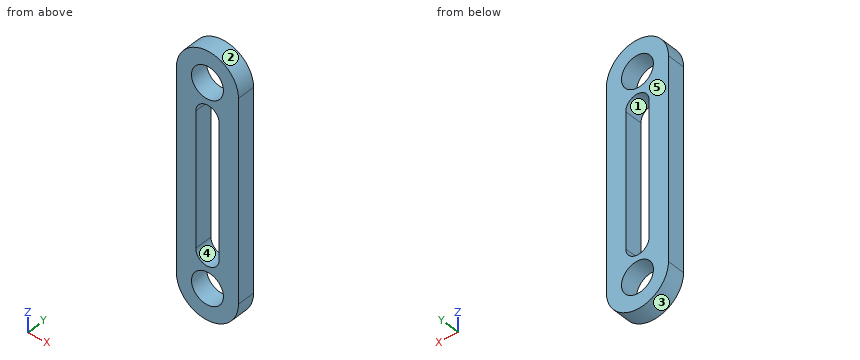
```python
from build123d import *

# Parameters (mm, degrees)
BOSS_EXTRUDE1_DEPTH             = 10
M16_CLEARANCE_HOLE1_D           = 17.5
M16_CLEARANCE_HOLE1_ON_FACE_2_D = 17.5


with BuildPart() as part:
    # Sketch1 → Boss-Extrude1 (new body)
    with BuildSketch(Plane(origin=(0, 0, 0), x_dir=(1, 0, 0), z_dir=(0, 1, 0))):
        with BuildLine():
            Line((17, 0), (17, -110))
            ThreePointArc((17, -110), (0, -127), (-17, -110))
            Line((-17, -110), (-17, 0))
            ThreePointArc((-17, 0), (0, 17), (17, 0))
        make_face()
        with BuildLine():
            Line((-6.39610115, -91.666666667), (-6.39610115, -18.333333333))
            ThreePointArc((-6.39610115, -18.333333333), (0, -11.937232183), (6.39610115, -18.333333333))
            Line((6.39610115, -18.333333333), (6.39610115, -91.666666667))
            ThreePointArc((6.39610115, -91.666666667), (0, -98.062767817), (-6.39610115, -91.666666667))
        make_face(mode=Mode.SUBTRACT)
    extrude(amount=BOSS_EXTRUDE1_DEPTH)

    # M16 Clearance Hole1 (through all)
    with Locations(Plane(origin=(0, 10, 110), x_dir=(0, 0, 1), z_dir=(0, 1, 0))):
        with Locations((0, 0), (-110, 0)):
            Hole(M16_CLEARANCE_HOLE1_D / 2)

    # M16 Clearance Hole1 on face 2 (through all)
    with Locations(Plane(origin=(0, 0, 0), x_dir=(0, 0, -1), z_dir=(0, -1, 0))):
        with Locations((0, 0)):
            Hole(M16_CLEARANCE_HOLE1_ON_FACE_2_D / 2)


solid = part.part
```
Can you work these out from the model? Positions are in its coordinate system, mm. Face numbers are marked on the shaded views. A direction names the side the tool comes from. Round coordinates to 2 decimals unless told otherwise and drop trailing zeros. Order: outer loops, then holes, each group sorted by start corner. A loop starts at its lowest first (then second) coordinate and runs counter-clockwise, first axis right, second up. Notation, with made-up numbers: (-7, -16.75) -> (1, -16.75) arc R8 ccw to (1, -5.75) -> close; hole circle Ø9 at (74, 58.25). An arc over 180 degrees is marked (long way). Return JSON: item names as keys, results as strings. Group by question number.
1. I need wall thicknesses on line 1 (X direction, y = 5.75, z = 52); line 2 (X direction, y = 7.75, z = 110); line 3 (Z direction, x = -4.5, y = 6). Which ranges of each line are inside material? Lowest first, please. Write a range as [from, to].
2. If we section it at A-A, the plane x = 0: Write out the boundary of the cut face in (y, z).
3. If we section it at B-B, the plane z = 89: Write out the boundary of the cut face in (x, y), then the cut area to 3 significant figures.
4. Which directions (+Z, -Z, +X, -X, +Y, -Y) give clear straight access to the entire face, cutting with the end or side of a thin tool? Please do the marked faces 1 and 2.
5. We'd pull the mould along Z, two halves only. Please class the marked faces 3, 4 and 5: released by +Z, released by -Z, zero draft, split by the parting line, or undercut.
6. If we section it at D-D, the plane x = 11.5: Write out the boundary of the cut face in (y, z), then the cut area to 3 significant figures.
7. If we section it at C-C, the plane y = 3.25: Write out the boundary of the cut face in (x, z).
Output values:
{
 "1": {"line 1": "[-17, -6.4], [6.4, 17]", "line 2": "[-17, -8.75], [8.75, 17]", "line 3": "[-16.39, -7.5], [7.5, 13.79], [96.21, 102.5], [117.5, 126.39]"},
 "2": {"outline": "(0, -17) -> (10, -17) -> (10, -8.75) -> (0, -8.75) -> close; (0, 8.75) -> (10, 8.75) -> (10, 11.94) -> (0, 11.94) -> close; (0, 98.06) -> (10, 98.06) -> (10, 101.25) -> (0, 101.25) -> close; (0, 118.75) -> (10, 118.75) -> (10, 127) -> (0, 127) -> close"},
 "3": {"outline": "(-17, 0) -> (-6.4, 0) -> (-6.4, 10) -> (-17, 10) -> close; (6.4, 0) -> (17, 0) -> (17, 10) -> (6.4, 10) -> close", "area": "212 mm²"},
 "4": {"face 1": "+Y, -Y", "face 2": "+Z, +Y, -Y"},
 "5": {"face 3": "released by -Z", "face 4": "undercut", "face 5": "zero draft"},
 "6": {"outline": "(0, -12.52) -> (10, -12.52) -> (10, 122.52) -> (0, 122.52) -> close", "area": "1,350 mm²"},
 "7": {"outline": "(-17, 0) arc R17 ccw to (17, 0) -> (17, 110) arc R17 ccw to (-17, 110) -> close; hole circle Ø17.5 at (0, 0); hole circle Ø17.5 at (0, 110); hole (-6.4, 18.33) arc R6.4 ccw to (6.4, 18.33) -> (6.4, 91.67) arc R6.4 ccw to (-6.4, 91.67) -> close"}
}
